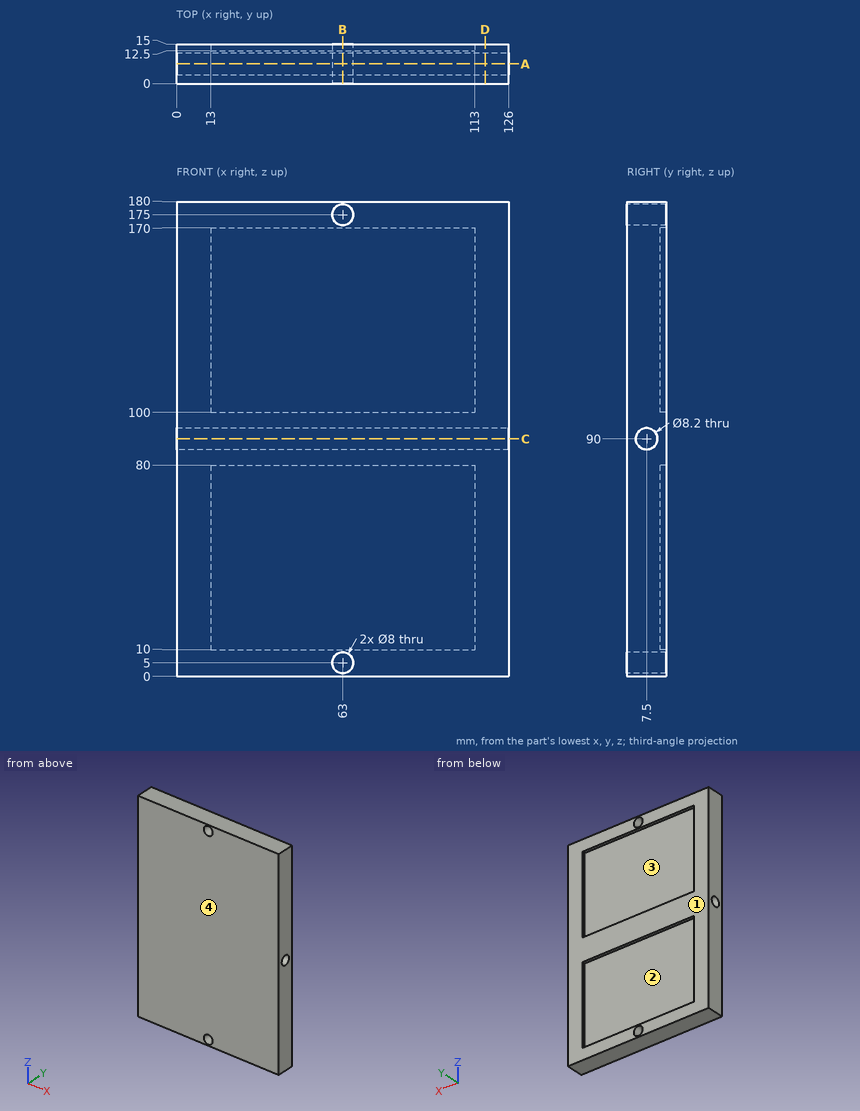
Here's the drawing with two shaded views (mm, measured from the low corner). I have some questions. A direction names the side the tool comes from. Round coordinates to 2 decimals unless told otherwise and drop trailing zeros. Write each loop counter-clockwise with the first axis right and the second up, starting at its lowest first coordinate (ties: lowest second). Pieces come first, ordered by that corner, then holes. Notation, with made-up numbers: M -24.5,75 L -17.5,75 A18 cw -17.5,88 Z; hole C -17.5,-37.5 d10. An arc over 180 degrees is marked long. Answer in a Markdown table with one row per item. Add a question column.
Q1. Will this pin go through, and if not, where does the flat tip stop? pin 1 Ø21 at (x, z) = (71, 55) entering from +Y.
Q2. Imagine slicing it at D-D (x = 117). Please give me the cut outline in (y, z), then the cut area to 3 significant figures.
Q3. Imagine slicing it at B-B (x = 63). Please give me the cut outline in (y, z).
Q4. If I drill on line 1 (Z direction, x = 58.5, y = 13.25); line 2 (Y direction, x = 80.5, z = 90); line 3 (Z direction, x = 64, y = 5.75), over which ranges is the centre line in solid material (lowest first)? Write a range as from..to.
Q5. Imagine slicing it at C-C (z = 90). Please give me the cut outline in (x, y), then the cut area to 3 significant figures.
Q6. On a 3-axis mill with a long thin cutter (end or side, diameter ignored), from which of +Z, -Z, +X, -X, +Y, -Y can I reach the whole of each face in a straight line? I mean the marked faces 1 and 2. Say none if no direction works.
Q7. Imagine slicing it at A-A (y = 7.5). Please give me the cut outline in (x, z).
Q8. If we mould it in two halves opening along Z, with no side actions, what happens to the marked faces 3 and 4? For each: +Z half, -Z half, draft (parallel to the pull), parting line (faces both ways), or undercut.
Values:
| question | item | result |
|---|---|---|
| 1 | pin 1 | y = 12.5 |
| 2 | outline | M 0,0 L 15,0 L 15,180 L 0,180 Z; hole C 7.5,90 d8.2 |
| 2 | area | 2,650 mm^2 |
| 3 | outline | M 0,0 L 15,0 L 15,1 L 0,1 Z; M 0,9 L 15,9 L 15,10 L 12.5,10 L 12.5,80 L 15,80 L 15,100 L 12.5,100 L 12.5,170 L 15,170 L 15,171 L 0,171 Z; M 0,179 L 15,179 L 15,180 L 0,180 Z; hole C 7.5,90 d8.2 |
| 4 | line 1 | 0..10, 80..100, 170..180 |
| 4 | line 2 | 0..3.4, 11.6..15 |
| 4 | line 3 | 0..1.13, 8.87..86.29, 93.71..171.13, 178.87..180 |
| 5 | outline | M 0,0 L 126,0 L 126,3.4 L 0,3.4 Z; M 0,11.6 L 126,11.6 L 126,15 L 0,15 Z |
| 5 | area | 857 mm^2 |
| 6 | face 1 | +Z, -Z, +X, -X, +Y |
| 6 | face 2 | +Y |
| 7 | outline | M 0,0 L 126,0 L 126,85.9 L 0,85.9 Z; M 0,94.1 L 126,94.1 L 126,180 L 0,180 Z; hole C 63,5 d8; hole C 63,175 d8 |
| 8 | face 3 | undercut |
| 8 | face 4 | draft |
